Here's how the part is built. I have some questions about the finished solid (model axes, mm). Face numbers are marked on the shaded views. Give positions to 0.01 mm unless a question says otherwise; leave off trailing zeros. Loops run counter-clockwise (first coordinate to the right, second up) from the corner with the lowest first, then second, coordinate; pieces in that order, holes last. Notation, with made-up numbers: (31, 45.5) - (85, 45.5) arc R19 cw to (85, 60.5) - close; hole circle Ø10 at (62.25, -8.75). An arc over 180 degrees is marked (long way). Return JSON: item names as keys, results as strings. Group by question number.
(1) If we section it at C-C (x = -29): Please give me the cut outline in (y, z), then the cut area to 3 significant figures.
(2) If we section it at B-B (z = -6): Please give me the cut outline in (x, y), then the cut area to 3 significant figures.
(3) If we mould it in two halves opening along Z, with no side actions, what happens to the marked faces 1 and 2? For each: released by +Z, released by -Z, zero draft, split by the parting line, or undercut.
(4) I need wall thicknesses on probe 1 along Z at (x, y) = (-29, -0.9); probe 2 along X at (y, z) = (-0.1, 13); probe 3 along Y at (x, z) = (-19.5, -20). Which ranges of each line are inside material? Lowest first, please. Write a range as [from, to].
(5) For P1, Ø13, axis at x = 7, z = -7, coming from the +Y side, with a flat end and sliding along its axis, tell me the tip position at first contact or that it passes through.
(6) If we section it at A-A (y = -0.5): Please give me the cut outline in (x, z), then the cut area to 3 significant figures.
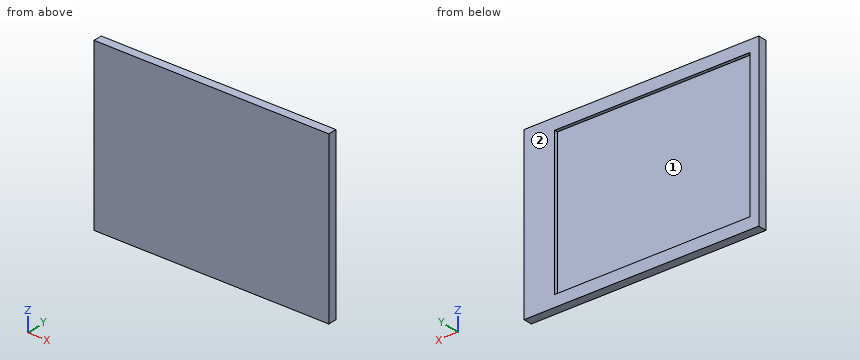
```python
from build123d import *

# Parameters (mm, degrees)
LCD_W               = 69.2
LCD_H               = 50
LCD_W_2             = 57.6
LCD_H_2             = 43.2
EXTRUDE_2_DEPTH     = 2.6
LCD_3_W             = 57.6
LCD_3_H             = 43.2
CUT_EXTRUDE_1_DEPTH = 1


with BuildPart() as part:
    # LCD → Extrude 2 (new body)
    with BuildSketch(Plane(origin=(0, 0, 0), x_dir=(1, 0, 0), z_dir=(0, 1, 0))):
        Rectangle(LCD_W, LCD_H)
        with Locations((-3.2, 0)):
            Rectangle(LCD_W_2, LCD_H_2, mode=Mode.SUBTRACT)
        with Locations((-3.2, 0)):
            Rectangle(LCD_W_2, LCD_H_2)
    extrude(amount=-EXTRUDE_2_DEPTH)

    # LCD_3 → Cut-Extrude 1 (cut)
    with BuildSketch(Plane(origin=(0, 0, 0), x_dir=(1, 0, 0), z_dir=(0, 1, 0))):
        with Locations((-3.2, 0)):
            Rectangle(LCD_3_W, LCD_3_H)
    extrude(amount=-CUT_EXTRUDE_1_DEPTH, mode=Mode.SUBTRACT)


solid = part.part
```
Values:
{
 "1": {"outline": "(-2.6, -25) - (0, -25) - (0, -21.6) - (-1, -21.6) - (-1, 21.6) - (0, 21.6) - (0, 25) - (-2.6, 25) - close", "area": "86.8 mm2"},
 "2": {"outline": "(-34.6, -2.6) - (34.6, -2.6) - (34.6, 0) - (25.6, 0) - (25.6, -1) - (-32, -1) - (-32, 0) - (-34.6, 0) - close", "area": "122 mm2"},
 "3": {"face 1": "undercut", "face 2": "zero draft"},
 "4": {"probe 1": "[-25, -21.6], [21.6, 25]", "probe 2": "[-34.6, -32], [25.6, 34.6]", "probe 3": "[-2.6, -1]"},
 "5": {"P1": "y = -1"},
 "6": {"outline": "(-34.6, -25) - (34.6, -25) - (34.6, 25) - (-34.6, 25) - close; hole (-32, -21.6) - (25.6, -21.6) - (25.6, 21.6) - (-32, 21.6) - close", "area": "972 mm2"}
}
